Part model, mm, in its own coordinate system. Round coordinates to 2 decimals unless told otherwise and drop trailing zeros. Write each loop counter-clockwise with the first axis right and the second up, starting at its lowest first coordinate (ties: lowest second). Pieces come first, ordered by that corner, then holes. Notation, with made-up numbers: M 7,-6 L 25,-6 A21 ccw 25,8 Z; hole C -22,-27 d1. An arc over 180 degrees is marked long. Answer as a JSON object with one key per item and string values. Group by question number.
1. Band-saw the part on A-A, the plane x = 4.5. Write the cut outline in (y, z).
2. Drill centre line: line 1 (Z direction, x = 3.5, y = -285.75). Where is it in solid material? Low to high. Write a range as from..to.
3. Drop flat-ended pins along their axis: pin 1 (6 mm diameter, centred on y = -152.4, z = 0, fed in from -X); pin 2 (3 mm diameter, centred on y = -196.85, z = 0, fed in from +X). Give the stop position or say it passes through.
4. Band-saw the part on B-B, the plane y = -285.75. Write the cut outline in (x, z), plus the area to 3 significant figures.
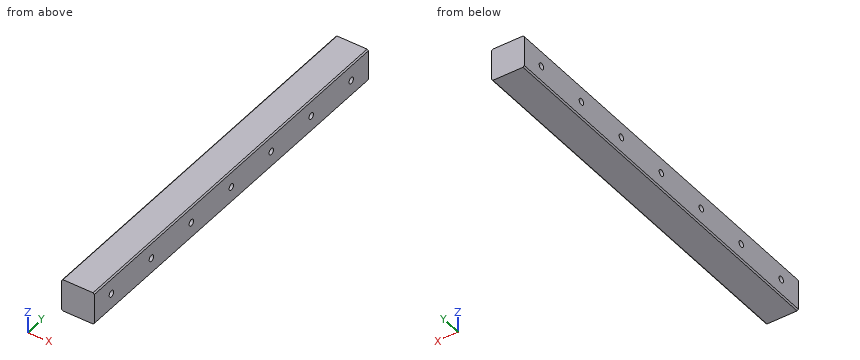
from build123d import *

# Parameters (mm, degrees)
F0_W     = 25.4
F0_H     = 25.4
F1_DEPTH = 304.8
F2_SIZE  = 1
F4_D     = 5


with BuildPart() as f1:
    # F0 (on Front) → F1 (new body)
    with BuildSketch(Plane.XZ):
        Rectangle(F0_W, F0_H)
    extrude(amount=F1_DEPTH)

    # F2
    f2_edges = [f1.edges().sort_by_distance(p)[0] for p in [
        (12.7, -152.4, 12.7),
        (12.7, -152.4, -12.7),
        (-12.7, -152.4, 12.7),
        (-12.7, -152.4, -12.7),
    ]]
    chamfer(f2_edges, length=F2_SIZE)

    # F4 (through all)
    with Locations(Plane.YZ.offset(12.7)):
        with Locations((-285.75, 0), (-241.3, 0), (-196.85, 0), (-152.4, 0), (-107.95, 0), (-63.5, 0), (-19.05, 0)):
            Hole(F4_D / 2)


solid = f1.part
Worked answers:
{
 "1": {"outline": "M -304.8,-12.7 L 0,-12.7 L 0,12.7 L -304.8,12.7 Z; hole C -285.75,0 d5; hole C -241.3,0 d5; hole C -196.85,0 d5; hole C -152.4,0 d5; hole C -107.95,0 d5; hole C -63.5,0 d5; hole C -19.05,0 d5"},
 "2": {"line 1": "z = -12.7..-2.5, 2.5..12.7"},
 "3": {"pin 1": "stops at x = -12.7", "pin 2": "passes through"},
 "4": {"outline": "M -12.7,-11.7 L -11.7,-12.7 L 11.7,-12.7 L 12.7,-11.7 L 12.7,-2.5 L -12.7,-2.5 Z; M -12.7,2.5 L 12.7,2.5 L 12.7,11.7 L 11.7,12.7 L -11.7,12.7 L -12.7,11.7 Z", "area": "516 mm^2"}
}
